Source: CAD feature listing. Evaluate the final solid. Frame: model axes, mm. Give positions to 0.01 mm unless a question says otherwise; leave off trailing zeros. Order: outer loops, then holes, each group sorted by start corner. A loop starts at its lowest first (then second) coordinate and runs counter-clockwise, first axis right, second up.
```python
from build123d import *

# Parameters (mm, degrees)
BOSS_EXTRUDE1_DEPTH            = 2.5
CHAMFER1_SIZE                  = 50
SKETCH4_W                      = 20
SKETCH4_H                      = 5
SKETCH4_R                      = 2
CUT_EXTRUDE1_DEPTH             = 5
SKETCH4_2_R                    = 2
CUT_EXTRUDE2_DEPTH             = 10
CRVPATTERN1_START              = -63.508529611
CRVPATTERN1_OUTLINE_W          = 20
CRVPATTERN1_OUTLINE_H          = 5
CRVPATTERN1_DEPTH              = 5
CRVPATTERN1_START_2            = -58.508529611
CRVPATTERN1_2_OUTLINE_R        = 2
CRVPATTERN1_2_DEPTH            = 5
CRVPATTERN1_START_3            = 58.508529611
CRVPATTERN1_3_OUTLINE_W        = 20
CRVPATTERN1_3_OUTLINE_H        = 5
CRVPATTERN1_3_DEPTH            = 5
CRVPATTERN1_START_4            = 53.508529611
CRVPATTERN1_4_OUTLINE_R        = 2
CRVPATTERN1_4_DEPTH            = 5
FILLET1_R                      = 10
CBORE_FOR_M2_SHCS1_D           = 2.4
CBORE_FOR_M2_SHCS1_CBORE_D     = 4.4
CBORE_FOR_M2_SHCS1_CBORE_DEPTH = 2


# Read off the part's stored shape, not the designer's step: CrvPattern1
with BuildPart() as part:
    # Sketch1 → Boss-Extrude1 (new, symmetric)
    with BuildSketch(Plane(origin=(0, 0, 0), x_dir=(1, 0, 0), z_dir=(0, 1, 0))):
        Polygon((110, -63.508529611), (0, 127.017059222), (-110, -63.508529611), align=None)
    extrude(amount=BOSS_EXTRUDE1_DEPTH, both=True)

    # Chamfer1
    chamfer1_edges = [part.edges().sort_by_distance(p)[0] for p in [
        (-110, 0, 63.508529611),
        (0, 0, -127.017059222),
        (110, 0, 63.508529611),
    ]]
    chamfer(chamfer1_edges, length=CHAMFER1_SIZE)

    # Sketch4 → Cut-Extrude1 (cut)
    with BuildSketch(Plane(origin=(4.375288244, 0, 63.508529611), x_dir=(-1, 0, 0), z_dir=(0, 0, -1))):
        with Locations((44.375288244, 0)):
            Rectangle(SKETCH4_W, SKETCH4_H)
        with Locations((39.375288244, 0)):
            Circle(SKETCH4_R, mode=Mode.SUBTRACT)
        with Locations((49.375288244, 0)):
            Circle(SKETCH4_R, mode=Mode.SUBTRACT)
    cut_extrude1 = extrude(amount=CUT_EXTRUDE1_DEPTH, mode=Mode.SUBTRACT)

    # Sketch4<2> → Cut-Extrude2 (cut)
    with BuildSketch(Plane(origin=(4.375288244, 0, 63.508529611), x_dir=(-1, 0, 0), z_dir=(0, 0, -1))):
        with Locations(Location((49.375288244, 0, 0), (0, 0, 180))):
            Circle(SKETCH4_2_R)
        with Locations(Location((39.375288244, 0, 0), (0, 0, 180))):
            Circle(SKETCH4_2_R)
    cut_extrude2 = extrude(amount=CUT_EXTRUDE2_DEPTH, mode=Mode.SUBTRACT)

    # Mirror1: Cut-Extrude1, Cut-Extrude2 across plane
    add(cut_extrude1.mirror(Plane(origin=(0, 0, 0), x_dir=(0, 0, 1), z_dir=(1, 0, 0))), mode=Mode.SUBTRACT)
    add(cut_extrude2.mirror(Plane(origin=(0, 0, 0), x_dir=(0, 0, 1), z_dir=(1, 0, 0))), mode=Mode.SUBTRACT)

    # CrvPattern1 outline → CrvPattern1 (cut)
    with BuildSketch(Plane(origin=(0, 0, 0), x_dir=(0.499999999999987, 0, -0.8660254037844463), z_dir=(0.8660254037844461, 0, 0.49999999999998707)).offset(CRVPATTERN1_START)):
        with Locations((-40, 0)):
            Rectangle(CRVPATTERN1_OUTLINE_W, CRVPATTERN1_OUTLINE_H)
        with Locations((40, 0)):
            Rectangle(CRVPATTERN1_OUTLINE_W, CRVPATTERN1_OUTLINE_H)
    extrude(amount=CRVPATTERN1_DEPTH, mode=Mode.SUBTRACT)

    # CrvPattern1 2 outline → CrvPattern1 2 (cut)
    with BuildSketch(Plane(origin=(0, 0, 0), x_dir=(0.499999999999987, 0, -0.8660254037844463), z_dir=(0.8660254037844461, 0, 0.49999999999998707)).offset(CRVPATTERN1_START_2)):
        with Locations((-35, 0)):
            Circle(CRVPATTERN1_2_OUTLINE_R)
        with Locations((-45, 0)):
            Circle(CRVPATTERN1_2_OUTLINE_R)
        with Locations((35, 0)):
            Circle(CRVPATTERN1_2_OUTLINE_R)
        with Locations((45, 0)):
            Circle(CRVPATTERN1_2_OUTLINE_R)
    extrude(amount=CRVPATTERN1_2_DEPTH, mode=Mode.SUBTRACT)

    # CrvPattern1 3 outline → CrvPattern1 3 (cut)
    with BuildSketch(Plane(origin=(0, 0, 0), x_dir=(0.500000000000001, 0, 0.866025403784438), z_dir=(0.866025403784438, 0, -0.500000000000001)).offset(CRVPATTERN1_START_3)):
        with Locations((-40, 0)):
            Rectangle(CRVPATTERN1_3_OUTLINE_W, CRVPATTERN1_3_OUTLINE_H)
        with Locations((40, 0)):
            Rectangle(CRVPATTERN1_3_OUTLINE_W, CRVPATTERN1_3_OUTLINE_H)
    extrude(amount=CRVPATTERN1_3_DEPTH, mode=Mode.SUBTRACT)

    # CrvPattern1 4 outline → CrvPattern1 4 (cut)
    with BuildSketch(Plane(origin=(0, 0, 0), x_dir=(0.500000000000001, 0, 0.866025403784438), z_dir=(0.866025403784438, 0, -0.500000000000001)).offset(CRVPATTERN1_START_4)):
        with Locations((-35, 0)):
            Circle(CRVPATTERN1_4_OUTLINE_R)
        with Locations((-45, 0)):
            Circle(CRVPATTERN1_4_OUTLINE_R)
        with Locations((35, 0)):
            Circle(CRVPATTERN1_4_OUTLINE_R)
        with Locations((45, 0)):
            Circle(CRVPATTERN1_4_OUTLINE_R)
    extrude(amount=CRVPATTERN1_4_DEPTH, mode=Mode.SUBTRACT)

    # Fillet1
    fillet1_edges = [part.edges().sort_by_distance(p)[0] for p in [
        (60, 0, 63.508529611),
        (-60, 0, 63.508529611),
        (-25, 0, -83.715789032),
        (-85, 0, 20.207259422),
        (25, 0, -83.715789032),
        (85, 0, 20.207259422),
    ]]
    fillet(fillet1_edges, radius=FILLET1_R)

    # CBORE for M2 SHCS1 (through all)
    with Locations(Plane(origin=(0, -2.5, 0), x_dir=(-1, 0, 0), z_dir=(0, -1, 0))):
        with Locations((-27.65, -10.65), (27.65, 10.65), (27.65, -10.65), (-27.65, 10.65)):
            CounterBoreHole(CBORE_FOR_M2_SHCS1_D / 2, CBORE_FOR_M2_SHCS1_CBORE_D / 2, CBORE_FOR_M2_SHCS1_CBORE_DEPTH)


solid = part.part
```
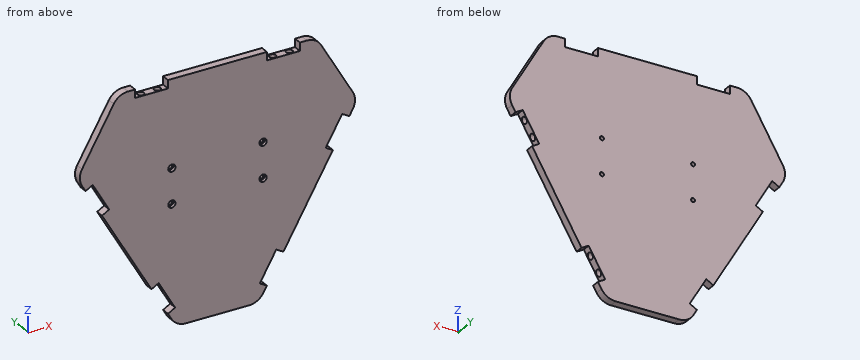
1) Material intervals for L1, parallel to X at y = -1.9, z = -10.65; L2, parallel to X at y = 0.25, z = -10.65; L3, parallel to Z at x = -27.65, y = 0.95, sorted ascending.
Report:
L1: x = -67.18 to -29.85, -25.45 to 25.45, 29.85 to 67.18
L2: x = -67.18 to -28.85, -26.45 to 26.45, 28.85 to 67.18
L3: z = -79.11 to -73.7, -65.89 to -11.85, -9.45 to 9.45, 11.85 to 63.51
2) Section query A-A, the plane x = 45. Return the cut outline in (y, z).
Report:
outline: (-2.5, -49.07) - (2.5, -49.07) - (2.5, 58.51) - (2, 58.51) - (2, 53.51) - (-2, 53.51) - (-2, 58.51) - (-2.5, 58.51) - close
3) Pin query (flat end, axial travel): pin 1 (2 mm diameter, centred on y = -1, z = 33.5, fed in from -X); pin 2 (1.3 mm diameter, centred on x = -28, z = 11.5, fed in from -Y); pin 3 (2.5 mm diameter, centred on x = -45, y = 0, fed in from +Z); pin 4 (2 mm diameter, centred on x = 27.65, z = -10.65, fed in from +Y). Return the tip coordinate at first contact, or that it passes through.
Report:
pin 1: stops at x = -77.9
pin 2: stops at y = -0.5
pin 3: stops at z = 53.51
pin 4: passes through
4) Section query B-B, the plane z = -41.5. Return the cut outline in (x, y), and give its area (3 significant figures).
Report:
outline: (-49.37, -2.5) - (49.37, -2.5) - (49.37, 2.5) - (-49.37, 2.5) - close
area: 494 mm2
5) Section query C-C, the plane y = 0.8. Count the separate pieces of the cut face and the enclosed holes in it, and give its area (3 significant figures).
Report:
separate pieces: 1
enclosed holes: 4
area: 16,800 mm2
6) Section query D-D, the plane x = -59.5. Return the cut outline in (y, z) (3 decimals), and give its area (3 significant figures).
Report:
outline: (-2.5, -23.96) - (2.5, -23.96) - (2.5, 62.005) - (-2.5, 62.005) - close
area: 430 mm2
